Geometry check sheet. Reference: the model listing, model coordinates, mm. Face numbers are marked on the shaded views. A direction names the side the tool comes from. Give positions to 0.01 mm unless a question says otherwise; leave off trailing zeros. Loops run counter-clockwise (first coordinate to the right, second up) from the corner with the lowest first, then second, coordinate; pieces in that order, holes last. Notation, with made-up numbers: (30, -13) -> (46, -13) arc R11 cw to (46, -6) -> close; hole circle Ø1 at (71.25, 18.5). An arc over 180 degrees is marked (long way). Write item = value, one per line.
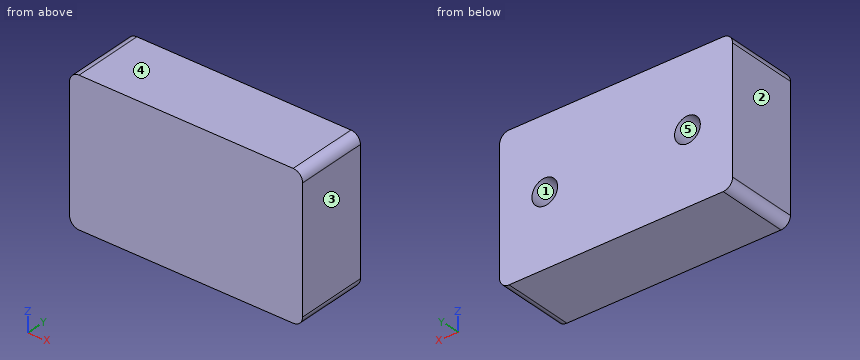
Autodesk Inventor part; units mm, degrees
ref_plane "YZ Plane" through (0, 0, 0) normal (1, 0, 0) x (0, 1, 0)
ref_plane "XZ Plane" through (0, 0, 0) normal (0, 1, 0) x (-1, 0, 0)
ref_plane "XY Plane" through (0, 0, 0) normal (0, 0, 1) x (1, 0, 0)
sketch "Boceto1" plane through (0, 0, 0) normal (0, 1, 0) x (-1, 0, 0)
  line L0 (-24.5, 15) -> (24.5, 15)
  line L1 (24.5, 15) -> (24.5, -15)
  line L2 (24.5, -15) -> (-24.5, -15)
  line L3 (-24.5, -15) -> (-24.5, 15)
  line L4 (-24.5, 15) -> (24.5, -15) construction
  line L5 (24.5, 15) -> (-24.5, -15) construction
  point P0 (0, 0)
  dimension "d0" = 49
  dimension "d1" = 30
extrude "Extrusión1" add sketch "Boceto1" along normal blind 15
sketch "Boceto2" plane through (0, 15, 0) normal (0, 1, 0) x (1, 0, 0)
  circle A0 centre (-15, 0) radius 2.7
  circle A1 centre (15, 0) radius 2.7
  line L0 (-24.5, 15) -> (-24.5, -15)
  line L1 (24.5, -15) -> (24.5, 15)
  point P0 (0, 0)
  dimension "d4" = 5.4
  dimension "d5" = 5.4
  dimension "d10" = 15
  dimension "d11" = 15
extrude "Extrusión2" cut sketch "Boceto2" against normal blind 7.5
fillet "Empalme1" radius 2 4 edges at (-24.5, 7.5, 15) (24.5, 7.5, 15) (24.5, 7.5, -15) (-24.5, 7.5, -15)
properties part number "Teeth"
Item 1: Section check C-C, the plane x = 15. Record the cut outline in (y, z).
Answer:
outline = (0, -15) -> (15, -15) -> (15, -2.7) -> (7.5, -2.7) -> (7.5, 2.7) -> (15, 2.7) -> (15, 15) -> (0, 15) -> close
Item 2: Section check B-B, the plane z = 0. Record the cut outline in (x, y), plus the area to 3 significant figures.
Answer:
outline = (-24.5, 0) -> (24.5, 0) -> (24.5, 15) -> (17.7, 15) -> (17.7, 7.5) -> (12.3, 7.5) -> (12.3, 15) -> (-12.3, 15) -> (-12.3, 7.5) -> (-17.7, 7.5) -> (-17.7, 15) -> (-24.5, 15) -> close
area = 654 mm^2
Item 3: Draft check along X on the marked faces 3, 4 and 5. Enter one of: +X half, -X half, draft (parallel to the pull), parting line (faces both ways), or undercut.
Answer:
face_3 = +X half
face_4 = draft
face_5 = undercut
Item 4: Thickness scan on L1, parallel to X at y = 11, z = 0; L2, parallel to Z at x = -15, y = 12.5; L3, parallel to X at y = 3.75, z = -13.5. Record the ranges inside material, lowest first. Write a range as [from, to].
Answer:
L1 = [-24.5, -17.7], [-12.3, 12.3], [17.7, 24.5]
L2 = [-15, -2.7], [2.7, 15]
L3 = [-24.44, 24.44]
Item 5: Tool access check on the marked faces 1 and 2. Record the directions out of +Z, -Z, +X, -X, +Y, -Y that give a thin tool (end or side, any length) a straight path to the whole face; none if there is none.
Answer:
face_1 = +Y
face_2 = +Z, -Z, -X, +Y, -Y
Item 6: Section check A-A, the plane y = 11.75. Record the cut outline in (x, z), plus the area to 3 significant figures.
Answer:
outline = (-24.5, -13) arc R2 ccw to (-22.5, -15) -> (22.5, -15) arc R2 ccw to (24.5, -13) -> (24.5, 13) arc R2 ccw to (22.5, 15) -> (-22.5, 15) arc R2 ccw to (-24.5, 13) -> close; hole circle Ø5.4 at (-15, 0); hole circle Ø5.4 at (15, 0)
area = 1,420 mm^2
Item 7: Gauge pin test, flat end, axial feed: pin 1 (3 mm diameter, centred on x = 15, z = 0, fed in from +Y). Record the tip position at first contact, or that the pin passes through.
Answer:
pin_1 = 7.5
